Geometry check sheet. Reference: the model listing, model coordinates, mm. Coordinates: 2 decimals unless noted, no trailing zeros. Write each loop counter-clockwise with the first axis right and the second up, starting at its lowest first coordinate (ties: lowest second). Pieces come first, ordered by that corner, then holes. Notation, with made-up numbers: (68.5, 30.5) -> (124.5, 30.5) arc R7 cw to (124.5, 42.5) -> close; hole circle Ø11 at (45, 66). An arc over 180 degrees is marked (long way). Answer in a Markdown table with one row per item. Add a question column.
1. Cross-section at B-B on z = 0. Record the cut outline in (x, y).
2. Cross-section at A-A on x = 0. Record the cut outline in (y, z).
3. Depth check by flat-ended pin: P1, Ø2.5, axis at y = 2.5, z = -70, coming from the +X side; P2, Ø2, axis at y = 6, z = 53.5, coming from the -X side; P3, Ø4, axis at y = 2, z = -16.5, coming from the +X side. Enter the tip coordinate at first touch or a pass-through.
4. Cross-section at C-C on y = 6.25. Record the cut outline in (x, z).
5. Scan lines: L1, parallel to X at y = 4.75, z = 0; L2, parallel to Z at x = 79.5, y = 6.75; L3, parallel to X at y = 6.75, z = -45. Record each from-to range of solid material in increasing order. Write a range as from..to.
6. Cross-section at D-D on z = -55. Record the cut outline in (x, y).
```python
from build123d import *

# Parameters (mm, degrees)
SKETCH1_R            = 125
SKETCH1_R_2          = 10
BOSS_EXTRUDE1_DEPTH  = 8
SKETCH2_W            = 16
SKETCH2_H            = 20
CUT_EXTRUDE1_DEPTH   = 10
LPATTERN1_COUNT      = 2
LPATTERN1_PITCH      = 144
LPATTERN1_COUNT_DIR2 = 2
LPATTERN1_PITCH_DIR2 = 100
SKETCH3_W            = 8
SKETCH3_H            = 20
CUT_EXTRUDE2_DEPTH   = 8


with BuildPart() as part:
    # Sketch1 → Boss-Extrude1 (new body)
    with BuildSketch(Plane(origin=(0, 0, 0), x_dir=(1, 0, 0), z_dir=(0, 1, 0))):
        with Locations(Location((0, 0, 0), (0, 0, 270))):
            Circle(SKETCH1_R)
        with Locations(Location((0, 0, 0), (0, 0, 270))):
            Circle(SKETCH1_R_2, mode=Mode.SUBTRACT)
    extrude(amount=BOSS_EXTRUDE1_DEPTH)

    # Sketch2 → Cut-Extrude1 (cut)
    with BuildSketch(Plane(origin=(0, 8, 0), x_dir=(1, 0, 0), z_dir=(0, 1, 0))):
        with Locations((-72, 50)):
            Rectangle(SKETCH2_W, SKETCH2_H)
    cut_extrude1 = extrude(amount=-CUT_EXTRUDE1_DEPTH, mode=Mode.SUBTRACT)

    # LPattern1: Cut-Extrude1 2 × 2
    with Locations(*[(i * LPATTERN1_PITCH, 0, j * LPATTERN1_PITCH_DIR2) for i in range(LPATTERN1_COUNT) for j in range(LPATTERN1_COUNT_DIR2) if (i, j) != (0, 0)]):
        add(cut_extrude1, mode=Mode.SUBTRACT)

    # Sketch3 → Cut-Extrude2 (cut)
    with BuildSketch(Plane(origin=(0, 8, 0), x_dir=(1, 0, 0), z_dir=(0, 1, 0))):
        with Locations((0, 70)):
            Rectangle(SKETCH3_W, SKETCH3_H)
    cut_extrude2 = extrude(amount=-CUT_EXTRUDE2_DEPTH, mode=Mode.SUBTRACT)

    # Mirror1: Cut-Extrude2 across plane
    add(cut_extrude2.mirror(Plane.XY), mode=Mode.SUBTRACT)


solid = part.part
```
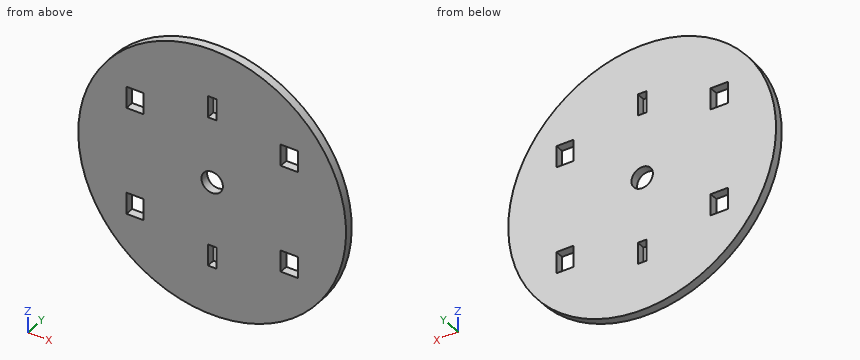
Results found:
| question | item | result |
|---|---|---|
| 1 | outline | (-125, 0) -> (-10, 0) -> (-10, 8) -> (-125, 8) -> close; (10, 0) -> (125, 0) -> (125, 8) -> (10, 8) -> close |
| 2 | outline | (0, -125) -> (8, -125) -> (8, -80) -> (0, -80) -> close; (0, -60) -> (8, -60) -> (8, -10) -> (0, -10) -> close; (0, 10) -> (8, 10) -> (8, 60) -> (0, 60) -> close; (0, 80) -> (8, 80) -> (8, 125) -> (0, 125) -> close |
| 3 | P1 | stops at x = 104.4 |
| 3 | P2 | stops at x = -113.44 |
| 3 | P3 | stops at x = 124.16 |
| 4 | outline | circle Ø250 at (0, 0); hole (-80, -60) -> (-64, -60) -> (-64, -40) -> (-80, -40) -> close; hole (-80, 40) -> (-64, 40) -> (-64, 60) -> (-80, 60) -> close; hole circle Ø20 at (0, 0); hole (-4, -80) -> (4, -80) -> (4, -60) -> (-4, -60) -> close; hole (-4, 60) -> (4, 60) -> (4, 80) -> (-4, 80) -> close; hole (64, -60) -> (80, -60) -> (80, -40) -> (64, -40) -> close; hole (64, 40) -> (80, 40) -> (80, 60) -> (64, 60) -> close |
| 5 | L1 | x = -125..-10, 10..125 |
| 5 | L2 | z = -96.46..-60, -40..40, 60..96.46 |
| 5 | L3 | x = -116.62..-80, -64..64, 80..116.62 |
| 6 | outline | (-112.25, 0) -> (-80, 0) -> (-80, 8) -> (-112.25, 8) -> close; (-64, 0) -> (64, 0) -> (64, 8) -> (-64, 8) -> close; (80, 0) -> (112.25, 0) -> (112.25, 8) -> (80, 8) -> close |
